Geometry: final body of the model. Coordinates: model frame, mm. Face numbers are marked on the shaded views. A direction names the side the tool comes from. Round coordinates to 2 decimals unless told otherwise and drop trailing zeros. Write each loop counter-clockwise with the first axis right and the second up, starting at its lowest first coordinate (ties: lowest second). Pieces come first, ordered by that corner, then holes. Notation, with made-up numbers: M 45,3 L 77,3 A16 cw 77,12 Z; hole C 86.25,-3.75 d9. An arc over 180 degrees is marked long. Use one line per item in the form item = value. Start each with the question number.
Item 1: Pin query (flat end, axial travel): pin 1 Ø10 at (y, z) = (171.5, -45) entering from +X; pin 2 Ø8 at (x, z) = (104, 318.5) entering from +Y; pin 3 Ø1 at (x, y) = (-27.5, 314.5) entering from +Z. Return the tip coordinate at first contact, or that it passes through.
Item 2: Section query D-D (y = 182). Return loops of the section in (x, z), and give its area (3 significant figures).
Item 3: Section query C-C (x = -253). Return loops of the section in (y, z), and give its area (3 significant figures).
Item 4: Ray query, probe 1 along Z at (x, y) = (-678.5, 181.5); probe 2 along X at (y, z) = (291, -185); probe 3 along X at (y, z) = (212, 31). Return the intervals inside material, ascending.
Item 5: Pull-direction query (X, two-part tool) for the marked faces 1, 2 and 3; classes: pulls with the +X half, pulls with the -X half, needs draft (parallel to the pull), parting line crosses it, or undercut.
Item 6: Reachability of the marked faces 4, 5 and 6 from +Z, -Z, +X, -X, +Y, -Y: full face, straight path, thin tool, end or side. Return the list, or none.
Item 7: Section query A-A (y = 301.5). Return loops of the section in (x, z), and give its area (3 significant figures).
Item 8: Section query B-B (z = -140.5). Return loops of the section in (x, y), and give its area (3 significant figures).
from build123d import *

# Parameters (mm, degrees)
EXTRUDE_THIN1_DEPTH = 215.9
SKETCH4_W           = 167.64
SKETCH4_H           = 728.98
BOSS_EXTRUDE3_DEPTH = 2.54
SKETCH6_W           = 1574.8
SKETCH6_H           = 1778
SKETCH6_W_2         = 1569.72
SKETCH6_H_2         = 1772.92
BOSS_EXTRUDE4_DEPTH = 368.3
BOSS_EXTRUDE6_DEPTH = 2.54
SKETCH9_W           = 1569.72
SKETCH9_H           = 2.54
CUT_EXTRUDE1_DEPTH  = 584.2


with BuildPart() as part:
    # Sketch1 → Extrude-Thin1 (new body)
    with BuildSketch(Plane(origin=(0, 0, 0), x_dir=(1, 0, 0), z_dir=(0, 1, 0))):
        Polygon((787.4, 889), (-787.4, 889), (-787.4, 469.9), (-622.3, 469.9), (-622.3, -254), (-787.4, -254), (-787.4, -889), (787.4, -889), (787.4, -254), (622.3, -254), (622.3, 469.9), (787.4, 469.9), align=None)
        Polygon((784.86, 886.46), (-784.86, 886.46), (-784.86, 472.44), (-619.76, 472.44), (-619.76, -256.54), (-784.86, -256.54), (-784.86, -886.46), (784.86, -886.46), (784.86, -256.54), (619.76, -256.54), (619.76, 472.44), (784.86, 472.44), align=None, mode=Mode.SUBTRACT)
    extrude(amount=EXTRUDE_THIN1_DEPTH)

    # Sketch4 → Boss-Extrude3 (add)
    with BuildSketch(Plane(origin=(0, 215.9, 0), x_dir=(1, 0, 0), z_dir=(0, 1, 0))):
        with Locations((-703.58, 107.95)):
            Rectangle(SKETCH4_W, SKETCH4_H)
        with Locations((703.58, 107.95)):
            Rectangle(SKETCH4_W, SKETCH4_H)
    extrude(amount=BOSS_EXTRUDE3_DEPTH)

    # Sketch6 → Boss-Extrude4 (add)
    with BuildSketch(Plane(origin=(0, 215.9, 0), x_dir=(1, 0, 0), z_dir=(0, 1, 0))):
        Rectangle(SKETCH6_W, SKETCH6_H)
        Rectangle(SKETCH6_W_2, SKETCH6_H_2, mode=Mode.SUBTRACT)
    extrude(amount=BOSS_EXTRUDE4_DEPTH)

    # Sketch8 → Boss-Extrude6 (add)
    with BuildSketch(Plane.XZ):
        Polygon((787.4, -889), (787.4, -469.9), (622.3, -469.9), (622.3, 254), (787.4, 254), (787.4, 889), (-787.4, 889), (-787.4, 254), (-622.3, 254), (-622.3, -469.9), (-787.4, -469.9), (-787.4, -889), align=None)
    extrude(amount=BOSS_EXTRUDE6_DEPTH)

    # Sketch9 → Cut-Extrude1 (cut)
    with BuildSketch(Plane(origin=(0, 584.2, 0), x_dir=(1, 0, 0), z_dir=(0, 1, 0))):
        with Locations((0, -887.73)):
            Rectangle(SKETCH9_W, SKETCH9_H)
    extrude(amount=-CUT_EXTRUDE1_DEPTH, mode=Mode.SUBTRACT)


solid = part.part
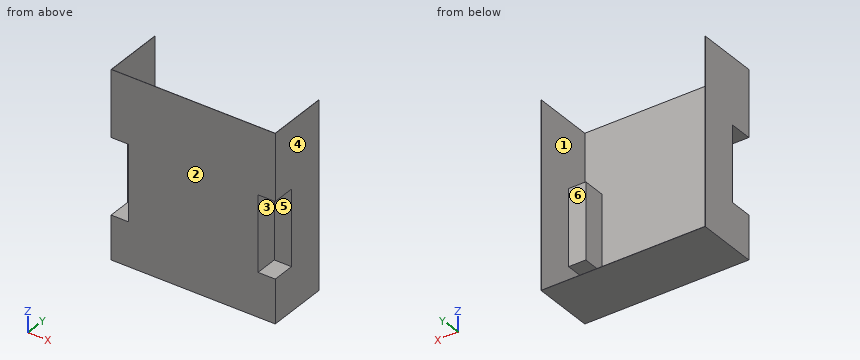
Working result:
q1.pin_1 = 622.3
q1.pin_2 = 0
q1.pin_3 = -886.46
q2.outline = M -787.4,-889 L 787.4,-889 L 787.4,-469.9 L 622.3,-469.9 L 622.3,254 L 787.4,254 L 787.4,889 L 784.86,889 L 784.86,256.54 L 619.76,256.54 L 619.76,-472.44 L 784.86,-472.44 L 784.86,-886.46 L -784.86,-886.46 L -784.86,-472.44 L -619.76,-472.44 L -619.76,256.54 L -784.86,256.54 L -784.86,889 L -787.4,889 L -787.4,254 L -622.3,254 L -622.3,-469.9 L -787.4,-469.9 Z
q2.area = 14,700 mm²
q3.outline = M -2.54,-889 L 584.2,-889 L 584.2,-886.46 L 0,-886.46 L 0,889 L -2.54,889 Z
q3.area = 6,000 mm²
q4.probe_1 = -889 to -886.46, -472.44 to -469.9, 254 to 256.54
q4.probe_2 = -787.4 to -784.86, 784.86 to 787.4
q4.probe_3 = -622.3 to -619.76, 619.76 to 622.3
q5.face_1 = undercut
q5.face_2 = needs draft
q5.face_3 = pulls with the +X half
q6.face_4 = +Z, -Z, +X, +Y, -Y
q6.face_5 = +X, -Y
q6.face_6 = +Z, +Y
q7.outline = M -787.4,-889 L 787.4,-889 L 787.4,889 L 784.86,889 L 784.86,-886.46 L -784.86,-886.46 L -784.86,889 L -787.4,889 Z
q7.area = 13,000 mm²
q8.outline = M -787.4,215.9 L -622.3,215.9 L -622.3,-2.54 L 622.3,-2.54 L 622.3,215.9 L 787.4,215.9 L 787.4,584.2 L 784.86,584.2 L 784.86,218.44 L 619.76,218.44 L 619.76,0 L -619.76,0 L -619.76,218.44 L -784.86,218.44 L -784.86,584.2 L -787.4,584.2 Z
q8.area = 6,970 mm²
